Input: part model. Units: mm. Frame: model coordinates. Face numbers are marked on the shaded views. A direction names the side the tool comes from. Coordinates: 2 decimals unless noted, no trailing zeros. Loops run counter-clockwise (first coordinate to the right, second up) from the corner with the lowest first, then second, coordinate; pieces in that order, holes last. Notation, with made-up numbers: (-17, 78.5) -> (13, 78.5) arc R14 cw to (13, 91.5) -> close; hole circle Ø7 at (88, 85). An arc over 180 degrees is marked (long way). Put each result on its own line as item: value. Start each with the question number.
1) Cut plane B-B (y = 2). Return the cut outline in (x, z).
2) Material intervals for L1, parallel to X at y = 0.7, z = -4.5; L2, parallel to Z at x = 22.25, y = 0.6; L3, parallel to X at y = 2.05, z = -4.5, sorted ascending.
3) Cut plane D-D (z = -1). Return the cut outline in (x, y), plus the area to 3 significant figures.
4) Cut plane A-A (x = 22.25). Return the cut outline in (y, z), plus the area to 3 significant figures.
5) Contact query for flat-ended pins moving along their axis: P1, Ø1.5, axis at x = 21, z = -1.5, coming from the +Y side; P2, Ø1.5, axis at x = 7, y = 4.5, coming from the +Z side. Output: stop coordinate, or through.
6) Cut plane C-C (x = 15.75). Return the cut outline in (y, z).
7) Set-up query: the marked faces 3 and 4. Return all of +Z, -Z, +X, -X, +Y, -Y with unobstructed straight access to the full face (end or side cutting, diameter ignored); none if empty.
8) Pull-direction query (Z, two-part tool) for the marked faces 1 and 2; classes: pulls with the +Z half, pulls with the -Z half, needs draft (parallel to the pull), parting line crosses it, or undercut.
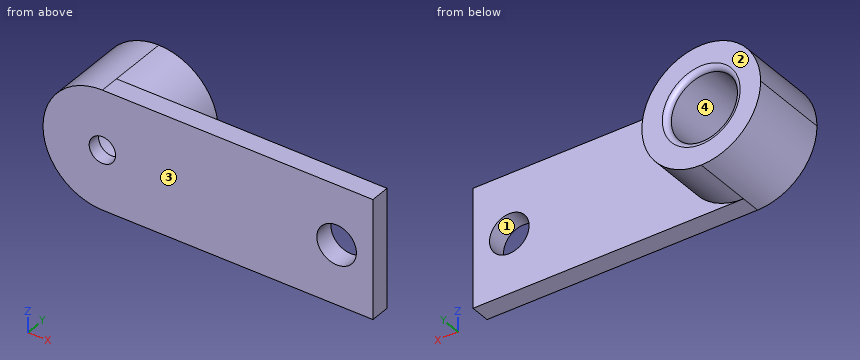
from build123d import *

# Parameters (mm, degrees)
SKETCH2_W               = 25
SKETCH2_H               = 9
BOSS_EXTRUDE3_DEPTH     = 6
SKETCH3_R               = 2.55
CUT_EXTRUDE1_DEPTH      = 5
CUT_EXTRUDE2_DEPTH      = 28.239676944
CUT_EXTRUDE2_DEPTH_BACK = 28.239676944
SKETCH4_R               = 1.5
SKETCH5_R               = 1.5
CUT_EXTRUDE3_DEPTH      = 4.5
CUT_EXTRUDE4_DEPTH      = 28.239676944
FILLET2_R               = 0.4
SKETCH8_R               = 1
CUT_EXTRUDE5_DEPTH      = 28.239676944


with BuildPart() as part:
    # Sketch2 → Boss-Extrude3 (new body)
    with BuildSketch(Plane(origin=(0, 0, 0), x_dir=(1, 0, 0), z_dir=(0, 1, 0))):
        with Locations((12.5, 4.5)):
            Rectangle(SKETCH2_W, SKETCH2_H)
    extrude(amount=BOSS_EXTRUDE3_DEPTH)

    # Sketch3 → Cut-Extrude1 (cut)
    with BuildSketch(Plane(origin=(0, 6, 0), x_dir=(1, 0, 0), z_dir=(0, 1, 0))):
        with Locations(Location((4.5, 4.5, 0), (0, 0, 270))):
            Circle(SKETCH3_R)
    extrude(amount=-CUT_EXTRUDE1_DEPTH, mode=Mode.SUBTRACT)

    # Sketch4 → Cut-Extrude2 (cut, two sides: drawn at the far end of the back side and taken through both)
    with BuildSketch(Plane(origin=(0, 6, 0), x_dir=(1, 0, 0), z_dir=(0, 1, 0)).offset(-CUT_EXTRUDE2_DEPTH_BACK)):
        with Locations(Location((22.25, 4.5, 0), (0, 0, 270))):
            Circle(SKETCH4_R)
    extrude(amount=CUT_EXTRUDE2_DEPTH + CUT_EXTRUDE2_DEPTH_BACK, mode=Mode.SUBTRACT)

    # Sketch5 → Cut-Extrude3 (cut)
    with BuildSketch(Plane(origin=(0, 6, 0), x_dir=(1, 0, 0), z_dir=(0, 1, 0))):
        with BuildLine():
            Line((25, 9), (4.5, 9))
            ThreePointArc((4.5, 9), (7.681980515, 7.681980515), (9, 4.5))
            ThreePointArc((9, 4.5), (7.681980515, 1.318019485), (4.5, 0))
            Line((4.5, 0), (25, 0))
            Line((25, 0), (25, 9))
        make_face()
        with Locations(Location((22.25, 4.5, 0), (0, 0, 270))):
            Circle(SKETCH5_R, mode=Mode.SUBTRACT)
    extrude(amount=-CUT_EXTRUDE3_DEPTH, mode=Mode.SUBTRACT)

    # Sketch6 → Cut-Extrude4 (cut, through all)
    with BuildSketch(Plane(origin=(0, 6, 0), x_dir=(1, 0, 0), z_dir=(0, 1, 0))):
        with BuildLine():
            ThreePointArc((0, 4.5), (1.318019485, 7.681980515), (4.5, 9))
            Line((4.5, 9), (0, 9))
            Line((0, 9), (0, 4.5))
        make_face()
        with BuildLine():
            ThreePointArc((4.5, 0), (1.318019485, 1.318019485), (0, 4.5))
            Line((0, 4.5), (0, 0))
            Line((0, 0), (4.5, 0))
        make_face()
    extrude(amount=-CUT_EXTRUDE4_DEPTH, mode=Mode.SUBTRACT)

    # Fillet2
    fillet2_edges = [part.edges().sort_by_distance(p)[0] for p in [
        (4.5, 6, -7.05),
    ]]
    fillet(fillet2_edges, radius=FILLET2_R)

    # Sketch8 → Cut-Extrude5 (cut, through all)
    with BuildSketch(Plane.XZ):
        with Locations(Location((4.5, -4.5, 0), (0, 0, 270))):
            Circle(SKETCH8_R)
    extrude(amount=-CUT_EXTRUDE5_DEPTH, mode=Mode.SUBTRACT)


solid = part.part
Results found:
1. outline: circle Ø9 at (4.5, -4.5); hole circle Ø5.1 at (4.5, -4.5)
2. L1: x = 0 to 3.5, 5.5 to 20.75, 23.75 to 25
2. L2: z = -9 to -6, -3 to 0
2. L3: x = 0 to 1.95, 7.05 to 9
3. outline: (1.67, 0) -> (25, 0) -> (25, 1.5) -> (7.33, 1.5) -> (7.33, 6) -> (1.67, 6) -> close
3. area: 60.4 mm2
4. outline: (0, -9) -> (1.5, -9) -> (1.5, -6) -> (0, -6) -> close; (0, -3) -> (1.5, -3) -> (1.5, 0) -> (0, 0) -> close
4. area: 9.00 mm2
5. P1: stops at y = 1.5
5. P2: stops at z = -0.35
6. outline: (0, -9) -> (1.5, -9) -> (1.5, 0) -> (0, 0) -> close
7. face 3: +Z, -Z, +X, -X, -Y
7. face 4: +Y
8. face 1: undercut
8. face 2: needs draft
